from build123d import *

# Parameters (mm, degrees)
BOSS_EXTRUDE1_DEPTH = 110
BOSS_EXTRUDE2_DEPTH = 3
LPATTERN1_COUNT     = 15
LPATTERN1_PITCH     = 7


with BuildPart() as part:
    # Sketch1 → Boss-Extrude1 (new body)
    with BuildSketch(Plane(origin=(0, 0, 0), x_dir=(1, 0, 0), z_dir=(0, 1, 0))):
        with BuildLine():
            Line((0, 0), (13, 0))
            ThreePointArc((13, 0), (38, 25), (63, 0))
            Line((63, 0), (78, 0))
            ThreePointArc((78, 0), (103, 25), (128, 0))
            Line((128, 0), (143, 0))
            ThreePointArc((143, 0), (168, 25), (193, 0))
            Line((193, 0), (208, 0))
            ThreePointArc((208, 0), (233, 25), (258, 0))
            Line((258, 0), (271, 0))
            Line((271, 0), (271, 65))
            ThreePointArc((271, 65), (268.071067812, 72.071067812), (261, 75))
            Line((261, 75), (10, 75))
            ThreePointArc((10, 75), (2.928932188, 72.071067812), (0, 65))
            Line((0, 65), (0, 0))
        make_face()
    extrude(amount=BOSS_EXTRUDE1_DEPTH)

    # Sketch2 → Boss-Extrude2 (add)
    with BuildSketch(Plane(origin=(0, 0, 0), x_dir=(1, 0, 0), z_dir=(0, 1, 0))):
        with BuildLine():
            Line((275, 0), (275, 65))
            ThreePointArc((275, 65), (270.899494937, 74.899494937), (261, 79))
            Line((261, 79), (10, 79))
            ThreePointArc((10, 79), (0.100505063, 74.899494937), (-4, 65))
            Line((-4, 65), (-4, 0))
            Line((-4, 0), (0, 0))
            Line((0, 0), (0, 65))
            ThreePointArc((0, 65), (2.928932188, 72.071067812), (10, 75))
            Line((10, 75), (261, 75))
            ThreePointArc((261, 75), (268.071067812, 72.071067812), (271, 65))
            Line((271, 65), (271, 0))
            Line((271, 0), (275, 0))
        make_face()
    boss_extrude2 = extrude(amount=BOSS_EXTRUDE2_DEPTH)

    # LPattern1: Boss-Extrude2 ×15
    with Locations(*[(0, i * LPATTERN1_PITCH, 0) for i in range(1, LPATTERN1_COUNT)]):
        add(boss_extrude2)


solid = part.part
Could you check a few things on this model? Use its own coordinates, in mm. A direction names the side the tool comes from. Give positions to 0.01 mm unless a question says otherwise; leave off trailing zeros. Answer in a Markdown table with one row per item. Add a question column.
Item 1: For faces 1 (the cylindrical face through (3.01, 88.97, -72.15)), 2 (the flat face through (271, 105, -32)), 3 (the flat face through (135, 54, 0)), which set-ups out of +Z, -Z, +X, -X, +Y, -Y let a thin tool reach every point of the face, with its end or its side?
Item 2: Imagine slicing it at A-A (z = -16). Count the separate pieces of the cut face and the enclosed holes in it, and give its area (3 significant figures).
Item 3: I'm going to push flat-ended pins straight in: P1, Ø1.2, axis at y = 68, z = -24.5, coming from the +X side; P2, Ø1.2, axis at x = 183, y = 11, coming from the -Z side; P3, Ø2, axis at y = 82.5, z = -41.5, coming from the -X side. Where does each tip first touch, or does it pass through?
Item 4: Please list where these lines run through material, in increasing order: probe 1 along X at (y, z) = (100, -17.5); probe 2 along X at (y, z) = (76.5, -13); probe 3 along X at (y, z) = (88.5, -42).
Item 5: We'd pull the mould along Y, two halves only. Please class faces 4 (the cylindrical face through (268.15, 53.97, -71.99)), 5 (the cylindrical face through (0.2, 85.5, -75)): pulls with the +Y half, pulls with the -Y half, needs draft (parallel to the pull), parting line crosses it, or undercut.
Result:
| question | item | result |
|---|---|---|
| 1 | face 1 | -Z, -X |
| 1 | face 2 | +Z, -Z, +X, +Y |
| 1 | face 3 | +Z, +X, -X, +Y, -Y |
| 2 | separate pieces | 5 |
| 2 | enclosed holes | 0 |
| 2 | area | 13,300 mm2 |
| 3 | P1 | x = 271 |
| 3 | P2 | z = -75 |
| 3 | P3 | x = 0 |
| 4 | probe 1 | -4 to 20.15, 55.85 to 85.15, 120.85 to 150.15, 185.85 to 215.15, 250.85 to 275 |
| 4 | probe 2 | 0 to 16.65, 59.35 to 81.65, 124.35 to 146.65, 189.35 to 211.65, 254.35 to 271 |
| 4 | probe 3 | 0 to 271 |
| 5 | face 4 | undercut |
| 5 | face 5 | needs draft |
